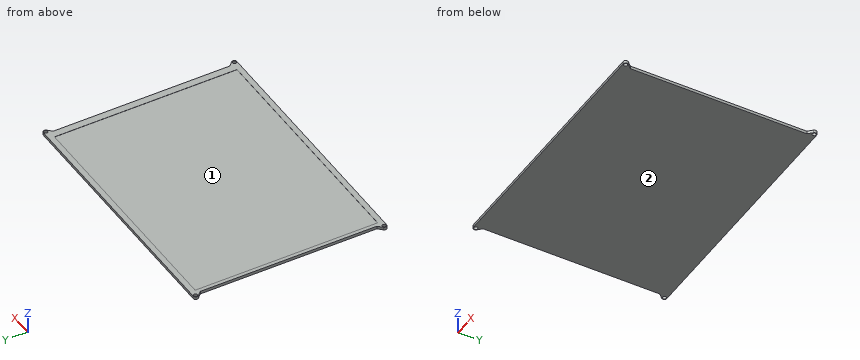
from build123d import *

# Parameters (mm, degrees)
CROQUIS1_W              = 209
CROQUIS1_H              = 160
CROQUIS1_R              = 1.5
SALIENTE_EXTRUIR1_DEPTH = 2.4
CROQUIS2_W              = 200
CROQUIS2_H              = 151
CORTAR_EXTRUIR1_DEPTH   = 0.2


with BuildPart() as part:
    # Croquis1 → Saliente-Extruir1 (new body)
    with BuildSketch(Plane.XY):
        Rectangle(CROQUIS1_W, CROQUIS1_H)
        with BuildLine():
            Line((-104.5, 73), (-104.5, 80))
            Line((-104.5, 80), (-106.5, 80))
            ThreePointArc((-106.5, 80), (-108.33829006, 78.787838597), (-107.948275862, 76.620689655))
            Line((-107.948275862, 76.620689655), (-104.5, 73))
        make_face()
        with Locations((-106.5, 78)):
            Circle(CROQUIS1_R, mode=Mode.SUBTRACT)
        with BuildLine():
            Line((106.5, 80), (104.5, 80))
            Line((104.5, 80), (104.5, 73))
            Line((104.5, 73), (107.948275862, 76.620689655))
            ThreePointArc((107.948275862, 76.620689655), (108.33829006, 78.787838597), (106.5, 80))
        make_face()
        with Locations((106.5, 78)):
            Circle(CROQUIS1_R, mode=Mode.SUBTRACT)
        with BuildLine():
            Line((107.948275862, -76.620689655), (104.5, -73))
            Line((104.5, -73), (104.5, -80))
            Line((104.5, -80), (106.5, -80))
            ThreePointArc((106.5, -80), (108.33829006, -78.787838597), (107.948275862, -76.620689655))
        make_face()
        with Locations((106.5, -78)):
            Circle(CROQUIS1_R, mode=Mode.SUBTRACT)
        with BuildLine():
            Line((-104.5, -80), (-104.5, -73))
            Line((-104.5, -73), (-107.948275862, -76.620689655))
            ThreePointArc((-107.948275862, -76.620689655), (-108.33829006, -78.787838597), (-106.5, -80))
            Line((-106.5, -80), (-104.5, -80))
        make_face()
        with Locations((-106.5, -78)):
            Circle(CROQUIS1_R, mode=Mode.SUBTRACT)
    extrude(amount=SALIENTE_EXTRUIR1_DEPTH)

    # Croquis2 → Cortar-Extruir1 (cut)
    with BuildSketch(Plane.XY.offset(2.4)):
        with Locations((-1.5, 0)):
            Rectangle(CROQUIS2_W, CROQUIS2_H)
    extrude(amount=-CORTAR_EXTRUIR1_DEPTH, mode=Mode.SUBTRACT)


solid = part.part
Could you check a few things on this model? Use its own coordinates, in mm. Face numbers are marked on the shaded views. Give positions to 0.01 mm unless a question says otherwise; leave off trailing zeros. Order: outer loops, then holes, each group sorted by start corner. A loop starts at its lowest first (then second) coordinate and runs counter-clockwise, first axis right, second up.
1. Will this pin go through, and if not, where does the flat tip stop? P1, Ø0.7, axis at y = -1.5, z = 1.5, coming from the -X side.
2. I need wall thicknesses on L1, parallel to X at y = -78, z = 1.15; L2, parallel to Y at x = 106.5, z = 1.15; L3, parallel to Z at x = -91.5, y = 38.5. Which ranges of each line are inside material? Lowest first, please.
3. Suppose I cut it at A-A (y = -34.5). List the corners of the cut face in (x, z) for me.
4. We'd pull the mould along Y, two halves only. Please class the marked faces 1 and 2: pulls with the +Y half, pulls with the -Y half, needs draft (parallel to the pull), parting line crosses it, or undercut.
5. Suppose I cut it at B-B (x = -73). List the corners of the cut face in (y, z) for me, plus the area to 3 significant figures.
Solved:
1. P1: stops at x = -104.5
2. L1: x = -108.5 to -108, -105 to 105, 108 to 108.5
2. L2: y = -80 to -79.5, -76.5 to -75.1, 75.1 to 76.5, 79.5 to 80
2. L3: z = 0 to 2.2
3. outline: (-104.5, 0) - (104.5, 0) - (104.5, 2.4) - (98.5, 2.4) - (98.5, 2.2) - (-101.5, 2.2) - (-101.5, 2.4) - (-104.5, 2.4) - close
4. face 1: undercut
4. face 2: needs draft
5. outline: (-80, 0) - (80, 0) - (80, 2.4) - (75.5, 2.4) - (75.5, 2.2) - (-75.5, 2.2) - (-75.5, 2.4) - (-80, 2.4) - close
5. area: 354 mm2
